Verification items for the finished model (mm, model axes). Give positions to 0.01 mm unless a question says otherwise; leave off trailing zeros. Order: outer loops, then holes, each group sorted by start corner. A loop starts at its lowest first (then second) coordinate and runs counter-clockwise, first axis right, second up. Notation, with made-up numbers: (-22.5, 89) -> (2.5, 89) arc R30 cw to (2.5, 115) -> close; hole circle Ø11 at (72, -13.5). An arc over 180 degrees is marked (long way). Write each question's results on one line, items separated by ' | '. Start each with the question number.
1. Cross-section at A-A, the plane x = -38.1. Enter the section's corners in (y, z).
2. Depth check by flat-ended pin: pin 1 Ø1.5 at (x, y) = (-62, -18) entering from -Z; pin 2 Ø8 at (x, z) = (-51.5, 39) entering from -Y; pin 3 Ø8 at (x, y) = (-9, 23.5) entering from +Z; pin 4 Ø5 at (x, z) = (-10, 52) entering from -Y. Enter the tip coordinate at first touch or a pass-through.
3. Cross-section at C-C, the plane z = 53.5. Enter the section's corners in (x, y).
4. Cross-section at B-B, the plane y = 0. Enter the section's corners in (x, z).
5. Material ranges on L1, parallel to Z at x = -68.5, y = 16; L2, parallel to Z at x = -54.5, y = 31; L3, parallel to X at y = 19, z = 96.5, recorded low to high. Write a range as from..to.
from build123d import *

# Parameters (mm, degrees)
F2_SIZE = 5.08
F3_SIZE = 5.08


with BuildPart() as f1:
    # F0 (on Front) → F1 (revolve)
    with BuildSketch(Plane.XZ):
        with BuildLine():
            Line((-38.1, 0), (0, 0))
            Line((0, 0), (0, 19.05))
            ThreePointArc((0, 19.05), (-6.35, 25.4), (0, 31.75))
            Line((0, 31.75), (0, 69.85))
            ThreePointArc((0, 69.85), (-6.35, 76.2), (0, 82.55))
            Line((0, 82.55), (0, 101.6))
            Line((0, 101.6), (-38.1, 101.6))
            Line((-38.1, 101.6), (-38.1, 0))
        make_face()
    revolve(axis=Axis((-38.1, 0, 50.8), (0, 0, 1)))

    # F2
    f2_edges = [f1.edges().sort_by_distance(p)[0] for p in [
        (-76.2, 0, 0),
    ]]
    chamfer(f2_edges, length=F2_SIZE)

    # F3
    f3_edges = [f1.edges().sort_by_distance(p)[0] for p in [
        (-76.2, 0, 101.6),
    ]]
    chamfer(f3_edges, length=F3_SIZE)


solid = f1.part
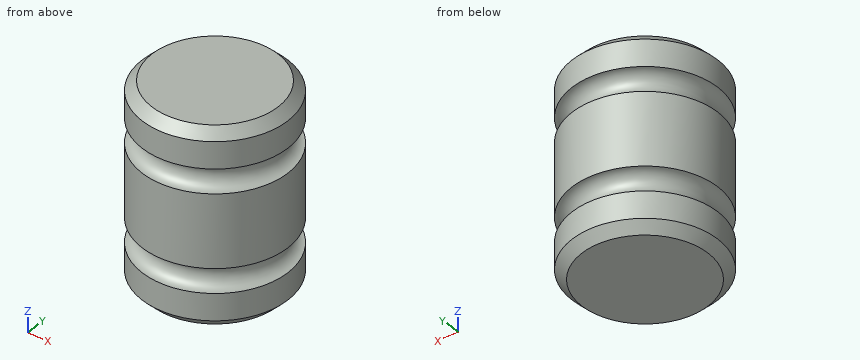
Results below:
1) outline: (-38.1, 5.08) -> (-33.02, 0) -> (33.02, 0) -> (38.1, 5.08) -> (38.1, 19.05) arc R6.35 cw to (38.1, 31.75) -> (38.1, 69.85) arc R6.35 cw to (38.1, 82.55) -> (38.1, 96.52) -> (33.02, 101.6) -> (-33.02, 101.6) -> (-38.1, 96.52) -> (-38.1, 82.55) arc R6.35 cw to (-38.1, 69.85) -> (-38.1, 31.75) arc R6.35 cw to (-38.1, 19.05) -> close
2) pin 1: stops at z = 0 | pin 2: stops at y = -36.92 | pin 3: stops at z = 101.22 | pin 4: stops at y = -28.22
3) outline: circle Ø76.2 at (-38.1, 0)
4) outline: (-76.2, 5.08) -> (-71.12, 0) -> (-5.08, 0) -> (0, 5.08) -> (0, 19.05) arc R6.35 cw to (0, 31.75) -> (0, 69.85) arc R6.35 cw to (0, 82.55) -> (0, 96.52) -> (-5.08, 101.6) -> (-71.12, 101.6) -> (-76.2, 96.52) -> (-76.2, 82.55) arc R6.35 cw to (-76.2, 69.85) -> (-76.2, 31.75) arc R6.35 cw to (-76.2, 19.05) -> close
5) L1: z = 1.33..20.27, 30.53..71.07, 81.33..100.27 | L2: z = 2.05..19.82, 30.98..70.62, 81.78..99.55 | L3: x = -71.12..-5.08
